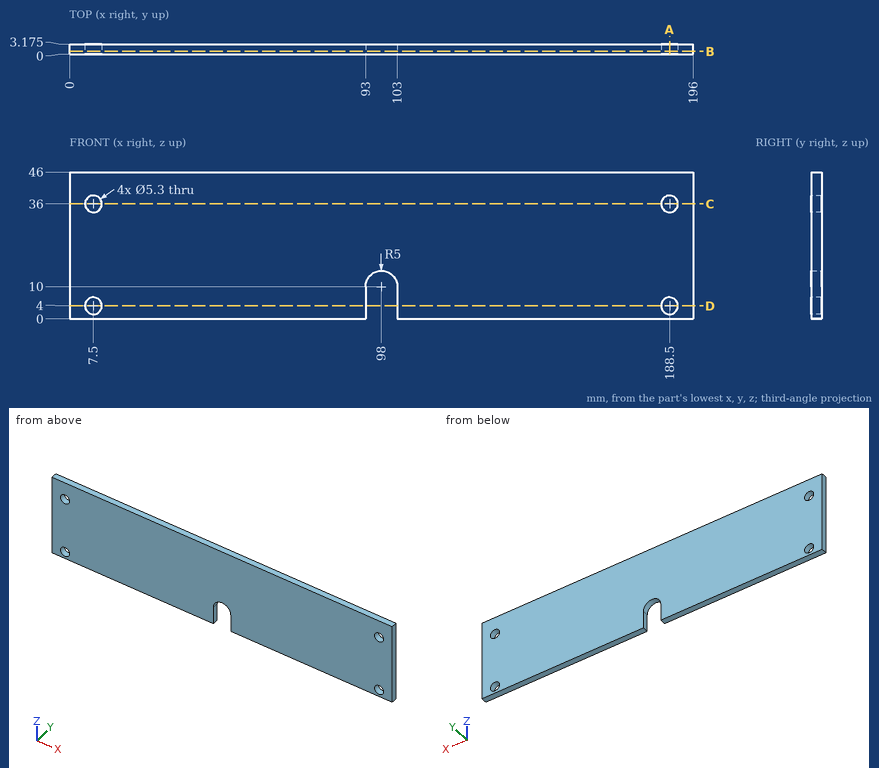
Source: three-view drawing plus pictorial views. Frame: mm from the lowest corner of the part. Round coordinates to 2 decimals unless told otherwise and drop trailing zeros. Order: outer loops, then holes, each group sorted by start corner. A loop starts at its lowest first (then second) coordinate and runs counter-clockwise, first axis right, second up. Notation, with made-up numbers: (52.5, 34.25) -> (82.5, 34.25) arc R24 ccw to (82.5, 48.25) -> close; hole circle Ø11 at (-27.5, 26.25). An arc over 180 degrees is marked (long way). Use CSV: the item, a comma, the result in double quotes. Start each with the question number.
1) Material intervals for line 1 along Z through (x, y) = (188.5, 2.5); line 2 along X through (y, z) = (2.3, 4); line 3 along X through (y, z) = (2.55, 36), sorted ascending. Write a range as from..to.
2) Section D-D (z = 4). Return the cut outline in (x, y) (3 decimals), and give its area (3 significant figures).
3) Section B-B (y = 0.85). Return the cut outline in (x, z).
4) Section A-A (x = 188.5). Return the cut outline in (y, z) (3 decimals).
5) Section C-C (z = 36). Return the cut outline in (x, y) (3 decimals).
Returned:
1,line 1,"z = 0..1.35, 6.65..33.35, 38.65..46"
1,line 2,"x = 0..4.85, 10.15..93, 103..185.85, 191.15..196"
1,line 3,"x = 0..4.85, 10.15..185.85, 191.15..196"
2,outline,"(0, 0) -> (4.85, 0) -> (4.85, 3.175) -> (0, 3.175) -> close; (10.15, 0) -> (93, 0) -> (93, 3.175) -> (10.15, 3.175) -> close; (103, 0) -> (185.85, 0) -> (185.85, 3.175) -> (103, 3.175) -> close; (191.15, 0) -> (196, 0) -> (196, 3.175) -> (191.15, 3.175) -> close"
2,area,"557 mm²"
3,outline,"(0, 0) -> (93, 0) -> (93, 10) arc R5 cw to (103, 10) -> (103, 0) -> (196, 0) -> (196, 46) -> (0, 46) -> close; hole circle Ø5.3 at (7.5, 4); hole circle Ø5.3 at (7.5, 36); hole circle Ø5.3 at (188.5, 4); hole circle Ø5.3 at (188.5, 36)"
4,outline,"(0, 0) -> (3.175, 0) -> (3.175, 1.35) -> (0, 1.35) -> close; (0, 6.65) -> (3.175, 6.65) -> (3.175, 33.35) -> (0, 33.35) -> close; (0, 38.65) -> (3.175, 38.65) -> (3.175, 46) -> (0, 46) -> close"
5,outline,"(0, 0) -> (4.85, 0) -> (4.85, 3.175) -> (0, 3.175) -> close; (10.15, 0) -> (185.85, 0) -> (185.85, 3.175) -> (10.15, 3.175) -> close; (191.15, 0) -> (196, 0) -> (196, 3.175) -> (191.15, 3.175) -> close"
